```python
from build123d import *

# Parameters (mm, degrees)
SKETCH_1_W               = 80
SKETCH_1_H               = 80
EXTRUDE_1_DEPTH          = 15
FILLET_1_R               = 20
SHELL_1_T                = -3
SKETCH_2_R               = 18
EXTRUDE_2_DEPTH          = 12
CUT_EXTRUDE_1_DEPTH      = 15
CUT_EXTRUDE_1_DEPTH_BACK = 15
SKETCH_2_3_R             = 15


with BuildPart() as part:
    # Sketch 1 → Extrude 1 (new body)
    with BuildSketch(Plane(origin=(0, 0, 0), x_dir=(1, 0, 0), z_dir=(0, 1, 0))):
        with Locations((40, 40)):
            Rectangle(SKETCH_1_W, SKETCH_1_H)
    extrude(amount=EXTRUDE_1_DEPTH)

    # Fillet 1
    fillet_1_edges = [part.edges().sort_by_distance(p)[0] for p in [
        (0, 7.5, 0),
        (0, 7.5, -80),
    ]]
    fillet(fillet_1_edges, radius=FILLET_1_R)

    # Shell 1
    shell_1_openings = [part.faces().sort_by_distance(p)[0] for p in [
        (40.979445098, 15, -40),
        (80, 7.5, -40),
    ]]
    offset(amount=SHELL_1_T, openings=shell_1_openings, kind=Kind.INTERSECTION)

    # Sketch 2 → Extrude 2 (add)
    with BuildSketch(Plane(origin=(0, 3, 0), x_dir=(1, 0, 0), z_dir=(0, 1, 0))):
        with Locations(Location((40, 40, 0), (0, 0, 270))):
            Circle(SKETCH_2_R)
    extrude(amount=EXTRUDE_2_DEPTH)

    # Sketch 2_3 → Cut-Extrude 1 (cut, two sides: drawn at the far end of the back side and taken through both)
    with BuildSketch(Plane(origin=(0, 3, 0), x_dir=(1, 0, 0), z_dir=(0, 1, 0)).offset(-CUT_EXTRUDE_1_DEPTH_BACK)):
        with Locations(Location((40, 40, 0), (0, 0, 270))):
            Circle(SKETCH_2_3_R)
    extrude(amount=CUT_EXTRUDE_1_DEPTH + CUT_EXTRUDE_1_DEPTH_BACK, mode=Mode.SUBTRACT)


solid = part.part
```
Input: part model. Units: mm. Frame: model coordinates. A direction names the side the tool comes from. Give positions to 0.01 mm unless a question says otherwise; leave off trailing zeros. Loops run counter-clockwise (first coordinate to the right, second up) from the corner with the lowest first, then second, coordinate; pieces in that order, holes last. Notation, with made-up numbers: M 81.5,72.5 L 126.5,72.5 A11 cw 126.5,78.5 Z; hole C 48,81 d1. An arc over 180 degrees is marked long. Answer as CSV lines item,"result". Start each with the question number.
1. Pin query (flat end, axial travel): P1, Ø5, axis at x = 38.5, z = -20.5, coming from the +Y side; P2, Ø4, axis at x = 59.5, z = -49.5, coming from the +Y side. Return the tip coordinate at first contact, or that it passes through.
2. Reachability of faces 1 (the face through (50, 7, -80)), 2 (the face through (50, 9, -77)), 3 (the face through (58, 3, -49)) from +Z, -Z, +X, -X, +Y, -Y: full face, straight path, thin tool, end or side. Return the list, or none.
3. Section D-D on y = 1.25. Return loops of the section in (x, z), plus the area to 3 significant figures.
4. Section B-B on y = 6. Return loops of the section in (x, z).
5. Pull-direction query (X, two-part tool) for faces 4 (the face through (50, 9, -3)), 5 (the face through (3, 9, -40)), 6 (the face through (5.703, 7.605, -6.014)); classes: released by +X, released by -X, zero draft, split by the parting line, or undercut.
6. Line query: L1, parallel to X at y = 5.25, z = -40; L2, parallel to Z at x = 39.5, y = 9.25; L3, parallel to Z at x = 20, y = 4.75. Output: solid intervals per line, ascending.
7. Section C-C on x = 40. Return loops of the section in (y, z).
8. Section A-A on z = -40. Return loops of the section in (x, y).
Computed values:
1,P1,"stops at y = 15"
1,P2,"stops at y = 3"
2,face 1,"-Z, +X, -X, +Y, -Y"
2,face 2,"+X, +Y"
2,face 3,"+Y"
3,outline,"M 0,-60 A20 ccw 20,-80 L 80,-80 L 80,0 L 20,0 A20 ccw 0,-20 Z; hole C 40,-40 d30"
3,area,"5,520 mm²"
4,outline,"M 0,-60 A20 ccw 20,-80 L 80,-80 L 80,-77 L 20,-77 A17 cw 3,-60 L 3,-20 A17 cw 20,-3 L 80,-3 L 80,0 L 20,0 A20 ccw 0,-20 Z; C 40,-40 d36; hole C 40,-40 d30"
5,face 4,"zero draft"
5,face 5,"undercut"
5,face 6,"released by -X"
6,L1,"x = 0 to 3, 22 to 25, 55 to 58"
6,L2,"z = -80 to -77, -57.99 to -54.99, -25.01 to -22.01, -3 to 0"
6,L3,"z = -80 to -77, -3 to 0"
7,outline,"M 0,-80 L 15,-80 L 15,-77 L 3,-77 L 3,-58 L 15,-58 L 15,-55 L 0,-55 Z; M 0,-25 L 15,-25 L 15,-22 L 3,-22 L 3,-3 L 15,-3 L 15,0 L 0,0 Z"
8,outline,"M 0,0 L 25,0 L 25,15 L 22,15 L 22,3 L 3,3 L 3,15 L 0,15 Z; M 55,0 L 80,0 L 80,3 L 58,3 L 58,15 L 55,15 Z"
